```python
from build123d import *

# Parameters (mm, degrees)
SHELL2_T = -3


with BuildPart() as part:
    # Sketch5 → Revolve11 (revolve)
    with BuildSketch(Plane.XY, mode=Mode.PRIVATE) as revolve11_sk:
        Polygon((-10.5, 0), (10.5, 0), (10.5, 12), (-5.5, 12), (-5.5, 15), (-10.5, 15), align=None)
    revolve(revolve11_sk.sketch.rotate(Axis((-10.5, 0, 0), (1, 0, 0)), 90), axis=Axis((-10.5, 0, 0), (1, 0, 0)))

    # Shell2
    shell2_openings = [part.faces().sort_by_distance(p)[0] for p in [
        (10.5, 0, 0),
        (-10.5, 0, 0),
    ]]
    offset(amount=SHELL2_T, openings=shell2_openings, kind=Kind.INTERSECTION)


solid = part.part
```
For this review, take the finished solid that the model builds, in its own axes (mm). A direction names the side the tool comes from. Give positions to 0.01 mm unless a question says otherwise; leave off trailing zeros. Write each loop counter-clockwise with the first axis right and the second up, starting at its lowest first coordinate (ties: lowest second). Pieces come first, ordered by that corner, then holes.
Item 1: Take a section at D-D (y = -9.5). Give the boundary of the cut face in (x, z), and give its area (3 significant figures).
Item 2: Insertion check: P1, Ø12, axis at x = -3, y = -11, coming from the -Z side; P2, Ø12, axis at x = 6.5, z = 11.5, coming from the -Y side; P3, Ø10, axis at x = -7.5, z = -9.5, coming from the +Y side. Each pin has a flat end and moves straight along its axis. Give the tip position at first contact, or say it passes through.
Item 3: Take a section at A-A (y = 0). Give the boundary of the cut face in (x, z), and give its area (3 significant figures).
Item 4: Take a section at C-C (x = 2.25). Give the boundary of the cut face in (y, z).
Item 5: Machinability: for faces 4 (the face through (10.5, -9, -2)), 5 (the face through (2.388, -3.604, 11.446)), 6 (the face through (-8.5, -9, -2)), which of the approach directions +Z, -Z, +X, -X, +Y, -Y give a long, thin tool a straight path to every point of the face, cutting with its end or side? Answer none if there is none.
Item 6: Wall thickness on probe 1 along Y at (x, z) = (-9.65, 0); probe 2 along Y at (x, z) = (4.5, 0); probe 3 along X at (y, z) = (0.5, -11.75): over which ranges is each line inside the solid? List them lowest first.
Item 7: The part is to be moulded in two halves that separate along Z. For faces 1 (the face through (-9.514, -3.604, 11.446)), 2 (the face through (-8.04, -12.65, 8.06)), 3 (the face through (-5.5, -10, 7)), say which applies: +Z half, -Z half, draft (parallel to the pull), parting line (faces both ways), or undercut.
Established:
1. outline: (-10.5, -11.61) - (-5.5, -11.61) - (-5.5, -7.33) - (10.5, -7.33) - (10.5, 7.33) - (-5.5, 7.33) - (-5.5, 11.61) - (-10.5, 11.61) - (-10.5, 7.33) - (-8.5, 7.33) - (-8.5, -7.33) - (-10.5, -7.33) - close
1. area: 321 mm2
2. P1: stops at z = -13.94
2. P2: stops at y = -10.67
2. P3: stops at y = 14.31
3. outline: (-10.5, -15) - (-5.5, -15) - (-5.5, -12) - (10.5, -12) - (10.5, -9) - (-8.5, -9) - (-8.5, -12) - (-10.5, -12) - close; (-10.5, 12) - (-8.5, 12) - (-8.5, 9) - (10.5, 9) - (10.5, 12) - (-5.5, 12) - (-5.5, 15) - (-10.5, 15) - close
3. area: 144 mm2
4. outline: circle Ø24 at (0, 0); hole circle Ø18 at (0, 0)
5. face 4: +Z, -Z, +X, +Y, -Y
5. face 5: +X
5. face 6: -X
6. probe 1: y = -15 to -12, 12 to 15
6. probe 2: y = -12 to -9, 9 to 12
6. probe 3: x = -8.5 to 10.5
7. face 1: undercut
7. face 2: parting line
7. face 3: draft
